Autodesk Inventor part; units mm, degrees
ref_plane "YZ Plane" through (0, 0, 0) normal (1, 0, 0) x (0, 1, 0)
ref_plane "XZ Plane" through (0, 0, 0) normal (0, 1, 0) x (-1, 0, 0)
ref_plane "XY Plane" through (0, 0, 0) normal (0, 0, 1) x (1, 0, 0)
sketch "スケッチ1" plane through (0, 0, 0) normal (0, 1, 0) x (-1, 0, 0)
  line L0 (0, 0) -> (400, 0)
  line L1 (400, 0) -> (400, -10)
  line L2 (400, -10) -> (0, -10)
  line L3 (0, -10) -> (0, 0)
  dimension "d0" = 400
  dimension "d1" = 10
extrude "押し出し1" add sketch "スケッチ1" along normal blind 10
sketch "スケッチ5" plane through (-400, 0, 0) normal (0, 0, 1) x (1, 0, 0)
  line L0 (400, 0) -> (400, 10)
  line L1 (0, 0) -> (0, 10)
  point P0 (385, 5)
  point P1 (15, 5)
  point P2 (400, 5)
  point P3 (400, 5)
  point P4 (0, 5)
  dimension "d13" = 15
  dimension "d14" = 15
hole "穴2" at (-15, 5, 0) at (-385, 5, 0) direction (0, 0, -1) diameter 3.1 end through all
properties part number "Yoko"
CAD build for the part. Positions are in the model's coordinates, mm. Coordinates: 2 decimals unless noted, no trailing zeros. Write each loop counter-clockwise with the first axis right and the second up, starting at its lowest first coordinate (ties: lowest second). Pieces come first, ordered by that corner, then holes.
(1) Drill centre lines: probe 1 along X at (y, z) = (4.75, -6); probe 2 along Y at (x, z) = (-15, -3.5). Where is each one in solid material? Low to high.
(2) Flat gauge pin, fed straight in: pin 1 (1.5 mm diameter, centred on x = -80.5, z = -5.5, fed in from -Y). Where does the tip first touch, or does it go through?
(3) Cut at A-A, the plane y = 5. List the corners of the cut face in (x, z), and give its area (3 significant figures).
Geometry says:
1. probe 1: x = -400 to -386.53, -383.47 to -16.53, -13.47 to 0
1. probe 2: y = 0 to 3.45, 6.55 to 10
2. pin 1: stops at y = 0
3. outline: (-400, -10) - (-386.55, -10) - (-386.55, 0) - (-400, 0) - close; (-383.45, -10) - (-16.55, -10) - (-16.55, 0) - (-383.45, 0) - close; (-13.45, -10) - (0, -10) - (0, 0) - (-13.45, 0) - close
3. area: 3,940 mm2
